Source: CAD feature listing. Evaluate the final solid. Frame: model axes, mm. Face numbers are marked on the shaded views. Coordinates: 2 decimals unless noted, no trailing zeros. Write each loop counter-clockwise with the first axis right and the second up, starting at its lowest first coordinate (ties: lowest second). Pieces come first, ordered by that corner, then holes. Notation, with made-up numbers: (-16, 8.25) - (32, 8.25) arc R6 ccw to (32, 12.25) - close; hole circle Ø8 at (-1.75, 27). An arc over 180 degrees is marked (long way). One line per question, with ' | ' between items.
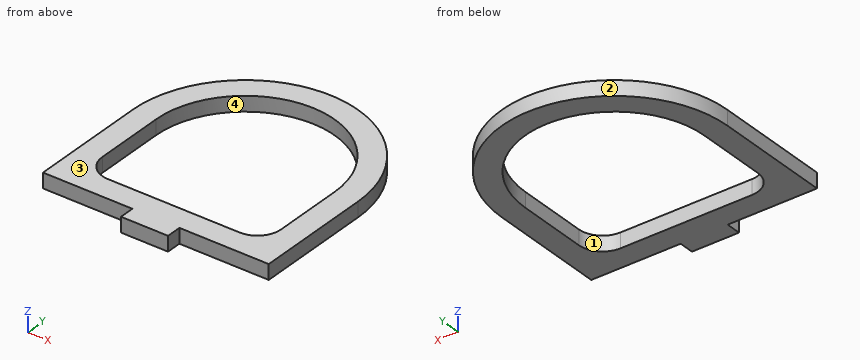
from build123d import *

# Parameters (mm, degrees)
F1_DEPTH = 3.175


with BuildPart() as f1:
    # F0 (on Top) → F1 (new body)
    with BuildSketch(Plane.XY):
        with BuildLine():
            Line((-25.744793, 17.416838), (-25.744793, -7.583162))
            Line((-25.744793, -7.583162), (-6.745631, -7.583162))
            Line((-6.745631, -7.583162), (-6.745631, -10.758162))
            Line((-6.745631, -10.758162), (3.254369, -10.758162))
            Line((3.254369, -10.758162), (3.254369, -7.583162))
            Line((3.254369, -7.583162), (22.253532, -7.583162))
            Line((22.253532, -7.583162), (22.253532, 17.416838))
            ThreePointArc((22.253532, 17.416838), (-1.745631, 41.416), (-25.744793, 17.416838))
        make_face()
        with BuildLine():
            ThreePointArc((-20.744793, 17.416838), (-1.745631, 36.416), (17.253532, 17.416838))
            Line((17.253532, 17.416838), (17.253532, 12.416838))
            Line((17.253532, 12.416838), (17.253532, 2.416838))
            ThreePointArc((17.253532, 2.416838), (15.789066, -1.118696), (12.253532, -2.583162))
            Line((12.253532, -2.583162), (3.254369, -2.583162))
            Line((3.254369, -2.583162), (-6.745631, -2.583162))
            Line((-6.745631, -2.583162), (-15.744793, -2.583162))
            ThreePointArc((-15.744793, -2.583162), (-19.280327, -1.118696), (-20.744793, 2.416838))
            Line((-20.744793, 2.416838), (-20.744793, 12.416838))
            Line((-20.744793, 12.416838), (-20.744793, 17.416838))
        make_face(mode=Mode.SUBTRACT)
    extrude(amount=F1_DEPTH)


solid = f1.part
Item 1: Cut plane B-B on x = -17.5. Return loops of the section in (y, z) (3 decimals), and give its area (3 significant figures).
Check sheet entries:
outline: (-7.583, 0) - (-2.265, 0) - (-2.265, 3.175) - (-7.583, 3.175) - close; (28.036, 0) - (35.521, 0) - (35.521, 3.175) - (28.036, 3.175) - close | area: 40.6 mm²
Item 2: Mould query, pull axis X, two halves, no side actions, for the marked faces 1, 2, 3 and 4. Classes: pulls with the +X half, pulls with the -X half, needs draft (parallel to the pull), parting line crosses it, or undercut.
Check sheet entries:
face 1: undercut | face 2: parting line crosses it | face 3: needs draft | face 4: undercut
Item 3: Pin query (flat end, axial travel): pin 1 Ø1 at (x, z) = (-11.5, 1) entering from -Y; pin 2 Ø1.6 at (y, z) = (-9, 2) entering from -X. Return the tip coordinate at first contact, or that it passes through.
Check sheet entries:
pin 1: y = -7.58 | pin 2: x = -6.75
Item 4: Cut plane A-A on y = 5. Return loops of the section in (x, z) (3 decimals).
Check sheet entries:
outline: (-25.745, 0) - (-20.745, 0) - (-20.745, 3.175) - (-25.745, 3.175) - close; (17.254, 0) - (22.254, 0) - (22.254, 3.175) - (17.254, 3.175) - close
Item 5: Ray query, line 1 along X through (y, z) = (12, 2.7); line 2 along Y through (x, z) = (-15, 0.4); line 3 along X through (y, z) = (32.5, 2.85). Return the intervals inside material, ascending. Write a range as [from, to].
Check sheet entries:
line 1: [-25.74, -20.74], [17.25, 22.25] | line 2: [-7.58, -2.58], [31.03, 37.42] | line 3: [-20.41, -13.3], [9.81, 16.92]
